```python
from build123d import *

# Parameters (mm, degrees)
SKETCH9_R                  = 38.1
BOSS_EXTRUDE2_DEPTH        = 3.556
BOSS_EXTRUDE3_START        = 3.556
SKETCH10_R                 = 38.1
BOSS_EXTRUDE3_DEPTH        = 3.556
F_3_4_0_3_DIAMETER_HOLE1_D = 7.62


with BuildPart() as part:
    # Sketch5 → Revolve1 (revolve)
    with BuildSketch(Plane(origin=(0, 0, 0), x_dir=(1, 0, 0), z_dir=(0, 1, 0)), mode=Mode.PRIVATE) as revolve1_sk:
        with BuildLine():
            Line((0, 0), (-38.1, 0))
            ThreePointArc((-38.1, 0), (-28.956, 9.144), (-38.1, 18.288))
            Line((-38.1, 18.288), (0, 18.288))
            Line((0, 18.288), (0, 0))
        make_face()
    revolve(revolve1_sk.sketch.rotate(Axis((0, 0, 0), (0, 0, -1)), 180), axis=Axis((0, 0, 0), (0, 0, -1)))

    # Sketch9 → Boss-Extrude2 (add)
    with BuildSketch(Plane.XY):
        Circle(SKETCH9_R)
    extrude(amount=BOSS_EXTRUDE2_DEPTH)

    # Sketch10 → Boss-Extrude3 (add)
    with BuildSketch(Plane(origin=(0, 0, -18.288), x_dir=(-1, 0, 0), z_dir=(0, 0, -1)).offset(BOSS_EXTRUDE3_START)):
        with Locations(Location((0, 0, 0), (0, 0, 180))):
            Circle(SKETCH10_R)
    extrude(amount=-BOSS_EXTRUDE3_DEPTH)

    # 3/4 (0.3) Diameter Hole1 (through all)
    with Locations(Plane.XY.offset(3.556)):
        with Locations((0, 0)):
            Hole(F_3_4_0_3_DIAMETER_HOLE1_D / 2)


solid = part.part
```
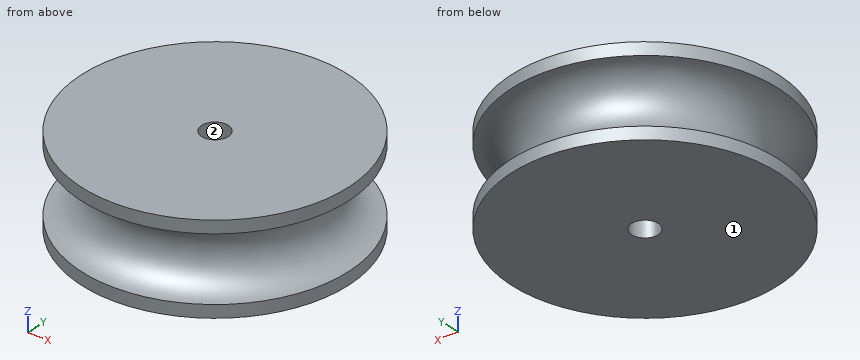
Geometry check sheet. Reference: the model listing, model coordinates, mm. Face numbers are marked on the shaded views. Coordinates: 2 decimals unless noted, no trailing zeros. Loops run counter-clockwise (first coordinate to the right, second up) from the corner with the lowest first, then second, coordinate; pieces in that order, holes last.
Item 1: Go/stop test with flat-tipped pins: pin 1 Ø8 at (y, z) = (5, -12.5) entering from -X; pin 2 Ø1.5 at (y, z) = (-15.5, -15) entering from +X; pin 3 Ø8 at (x, z) = (-25, -18.5) entering from -Y. Record where each tip stops, or that it passes through.
Item 2: Sectioned sample at D-D, the plane z = -6.25. Record the boundary of the cut face in (x, y), then the cut area to 3 significant figures.
Item 3: Release check for a two-part mould opening along X. For the marked faces 1 and 2 record: released by +X, released by -X, zero draft, split by the parting line, or undercut.
Item 4: Sectioned sample at A-A, the plane x = 0. Record the boundary of the cut face in (y, z), then the cut area to 3 significant figures.
Item 5: Thickness scan on line 1 (Y direction, x = 0, z = -4.5); line 2 (Z direction, x = -32, y = 12.5); line 3 (Y direction, x = 0, z = -5.5). Record the ranges inside material, lowest first.
Item 6: Sectioned sample at C-C, the plane z = 1.25. Record the boundary of the cut face in (x, y).
Check result:
1. pin 1: stops at x = -32.32
1. pin 2: stops at x = 27.83
1. pin 3: stops at y = -31.79
2. outline: circle Ø58.85 at (0, 0); hole circle Ø7.62 at (0, 0)
2. area: 2,670 mm2
3. face 1: zero draft
3. face 2: undercut
4. outline: (-38.1, -21.84) - (-3.81, -21.84) - (-3.81, 3.56) - (-38.1, 3.56) - (-38.1, 0) arc R9.14 cw to (-38.1, -18.29) - close; (3.81, -21.84) - (38.1, -21.84) - (38.1, -18.29) arc R9.14 cw to (38.1, 0) - (38.1, 3.56) - (3.81, 3.56) - close
4. area: 1,480 mm2
5. line 1: y = -30.22 to -3.81, 3.81 to 30.22
5. line 2: z = -21.84 to -17.49, -0.8 to 3.56
5. line 3: y = -29.71 to -3.81, 3.81 to 29.71
6. outline: circle Ø76.2 at (0, 0); hole circle Ø7.62 at (0, 0)
